from build123d import *

# Parameters (mm, degrees)
SKETCH_1_R          = 52.5
SKETCH_1_R_2        = 48.5
EXTRUDE_1_DEPTH     = 3.2
SKETCH_2_R          = 51.5
CUT_EXTRUDE_1_DEPTH = 2.2
SKETCH_3_R          = 1.25
EXTRUDE_2_DEPTH     = 1.1
EXTRUDE_3_DEPTH     = 1.1
SKETCH_5_R          = 0.7
CUT_EXTRUDE_2_DEPTH = 75.315139776
SKETCH_6_R          = 1.5
CUT_EXTRUDE_3_DEPTH = 0.7
FILLET_1_R          = 0.5
CHAMFER_1_SIZE      = 0.3
CHAMFER_1_SIZE2     = 0.357526078


with BuildPart() as part:
    # 草图1 → 凸台-拉伸1 (new body)
    with BuildSketch(Plane(origin=(0, 0, 0), x_dir=(1, 0, 0), z_dir=(0, 1, 0))):
        with Locations(Location((0, 0, 0), (0, 0, 270))):
            Circle(SKETCH_1_R)
        with Locations(Location((0, 0, 0), (0, 0, 270))):
            Circle(SKETCH_1_R_2, mode=Mode.SUBTRACT)
    extrude(amount=EXTRUDE_1_DEPTH)

    # 草图2 → 切除-拉伸1 (cut)
    with BuildSketch(Plane(origin=(0, 3.2, 0), x_dir=(1, 0, 0), z_dir=(0, 1, 0))):
        with Locations(Location((0, 0, 0), (0, 0, 270))):
            Circle(SKETCH_2_R)
    extrude(amount=-CUT_EXTRUDE_1_DEPTH, mode=Mode.SUBTRACT)

    # 草图3 → 凸台-拉伸2 (add)
    with BuildSketch(Plane(origin=(0, 1, 0), x_dir=(1, 0, 0), z_dir=(0, 1, 0))):
        with Locations((-43.734282891, -25.25)):
            Circle(SKETCH_3_R)
        with Locations((43.734282891, -25.25)):
            Circle(SKETCH_3_R)
        with Locations((0, 50.5)):
            Circle(SKETCH_3_R)
    extrude(amount=EXTRUDE_2_DEPTH)

    # 草图4 → 凸台-拉伸3 (add)
    with BuildSketch(Plane(origin=(0, 1, 0), x_dir=(1, 0, 0), z_dir=(0, 1, 0))):
        with BuildLine():
            ThreePointArc((-44.974169566, -25.09131467), (-44.774871009, -24.557413277), (-44.359282891, -24.167468245))
            Line((-44.359282891, -24.167468245), (-45.225308295, -24.667468245))
            Line((-45.225308295, -24.667468245), (-44.600307976, -25.750000552))
            ThreePointArc((-44.600307976, -25.750000552), (-44.788449666, -25.4213449), (-44.974169566, -25.09131467))
        make_face()
        with BuildLine():
            Line((-43.975308295, -26.832531755), (-43.109282891, -26.332531755))
            ThreePointArc((-43.109282891, -26.332531755), (-43.654779254, -26.497469106), (-44.216800701, -26.403116023))
            ThreePointArc((-44.216800701, -26.403116023), (-44.409754992, -26.077263307), (-44.600307976, -25.750000552))
            Line((-44.600307976, -25.750000552), (-43.975308295, -26.832531755))
        make_face()
        with BuildLine():
            Line((-1.59e-07, 51.5), (-1.25, 51.5))
            Line((-1.25, 51.5), (-1.25, 50.5))
            ThreePointArc((-1.25, 50.5), (-1.120091755, 51.054882384), (-0.757368864, 51.494430693))
            ThreePointArc((-0.757368864, 51.494430693), (-0.37869475, 51.498607654), (-1.59e-07, 51.5))
        make_face()
        with BuildLine():
            Line((1.25, 51.5), (-1.59e-07, 51.5))
            ThreePointArc((-1.59e-07, 51.5), (0.378694591, 51.498607655), (0.757368864, 51.494430693))
            ThreePointArc((0.757368864, 51.494430693), (1.120091755, 51.054882384), (1.25, 50.5))
            Line((1.25, 50.5), (1.25, 51.5))
        make_face()
        with BuildLine():
            Line((45.225308295, -24.667468245), (44.359282891, -24.167468245))
            ThreePointArc((44.359282891, -24.167468245), (44.774871009, -24.557413277), (44.974169566, -25.09131467))
            ThreePointArc((44.974169566, -25.09131467), (44.788449793, -25.421344676), (44.600308233, -25.750000108))
            Line((44.600308233, -25.750000108), (45.225308295, -24.667468245))
        make_face()
        with BuildLine():
            ThreePointArc((44.216800701, -26.403116023), (43.654779254, -26.497469107), (43.109282891, -26.332531755))
            Line((43.109282891, -26.332531755), (43.975308295, -26.832531755))
            Line((43.975308295, -26.832531755), (44.600308233, -25.750000108))
            ThreePointArc((44.600308233, -25.750000108), (44.409755121, -26.077263086), (44.216800701, -26.403116023))
        make_face()
    extrude(amount=EXTRUDE_3_DEPTH)

    # 草图5 → 切除-拉伸2 (cut, through all)
    with BuildSketch(Plane(origin=(0, 3.2, 0), x_dir=(1, 0, 0), z_dir=(0, 1, 0))):
        with Locations(Location((0, 50.5, 0), (0, 0, 270))):
            Circle(SKETCH_5_R)
        with Locations(Location((-43.734282891, -25.25, 0), (0, 0, 270))):
            Circle(SKETCH_5_R)
        with Locations(Location((43.734282891, -25.25, 0), (0, 0, 270))):
            Circle(SKETCH_5_R)
    extrude(amount=-CUT_EXTRUDE_2_DEPTH, mode=Mode.SUBTRACT)

    # 草图6 → 切除-拉伸3 (cut)
    with BuildSketch(Plane.XZ):
        with Locations(Location((-43.734282891, 25.25, 0), (0, 0, 270))):
            Circle(SKETCH_6_R)
        with Locations(Location((0, -50.5, 0), (0, 0, 270))):
            Circle(SKETCH_6_R)
        with Locations(Location((43.734282891, 25.25, 0), (0, 0, 270))):
            Circle(SKETCH_6_R)
    extrude(amount=-CUT_EXTRUDE_3_DEPTH, mode=Mode.SUBTRACT)

    # 圆角1
    fillet_1_edges = [part.edges().sort_by_distance(p)[0] for p in [
        (0, 0, -52.5),
        (-43.962168838, 1.55, 26.824945686),
        (-45.212168838, 1.55, 24.659882176),
        (-1.25, 1.55, -51.484827862),
        (1.25, 1.55, -51.484827862),
        (45.212168838, 1.55, 24.659882176),
        (43.962168838, 1.55, 26.824945686),
    ]]
    fillet(fillet_1_edges, radius=FILLET_1_R - 0.0001)  # a hair under: the kernel refuses the full size

    # 倒角1
    chamfer_1_edges = [part.edges().sort_by_distance(p)[0] for p in [
        (0, 0, -48.5),
    ]]
    chamfer_1_side = [part.faces().sort_by_distance(p)[0] for p in [
        (0, 0.5, -48.5),
    ]]
    chamfer(chamfer_1_edges, length=CHAMFER_1_SIZE, length2=CHAMFER_1_SIZE2, reference=chamfer_1_side[0])


solid = part.part
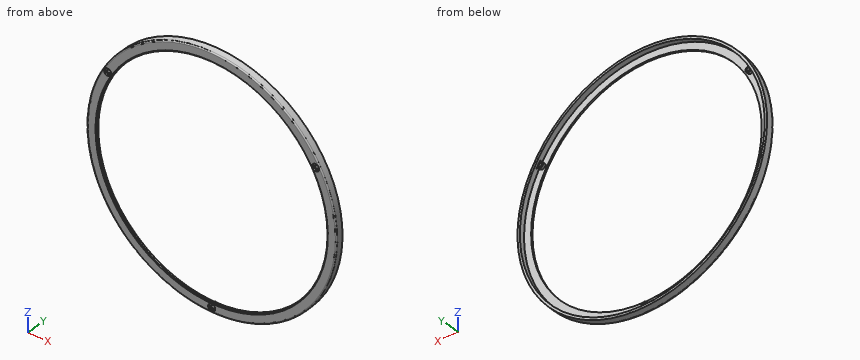
Read the model definition and answer for the solid it produces. Units are mm, in the model's axes. Coordinates: 2 decimals unless noted, no trailing zeros. Loops run counter-clockwise (first coordinate to the right, second up) from the corner with the lowest first, then second, coordinate; pieces in that order, holes last. Notation, with made-up numbers: (43, -16) - (92, -16) arc R25 ccw to (92, 5) - close; hole circle Ø5 at (61, 25.5). An arc over 180 degrees is marked (long way). Answer in a Markdown table with one row per item.
Q1. Given P1, Ø1.8, axis at x = 0.5, z = -50.5, coming from the +Y side; P2, Ø1, axis at y = 1, z = -24.5, coming from the -X side; P3, Ø1.5, axis at y = 0.5, z = -9.5, coming from the -X side, each flat-ended and moving along its own axis, determine where each tip first touches the part or whether it passes through.
Here are the results:
| item | result |
|---|---|
| P1 | stops at y = 2.1 |
| P2 | stops at x = -46.69 |
| P3 | stops at x = -51.77 |
Q2. Find section B-B on y = 1.6. Write down the section's boundary in (x, z).
Here are the results:
| item | result |
|---|---|
| outline | circle Ø105 at (0, 0); hole (-45.46, 24.2) arc R51.5 ccw to (-1.77, -51.47) arc R0.5 ccw to (-1.25, -50.97) - (-1.25, -50.5) arc R1.25 cw to (1.25, -50.5) - (1.25, -50.97) arc R0.5 ccw to (1.77, -51.47) arc R51.5 ccw to (45.46, 24.2) arc R0.5 ccw to (44.77, 24.4) - (44.36, 24.17) arc R1.25 cw to (43.11, 26.33) - (43.52, 26.57) arc R0.5 ccw to (43.69, 27.27) arc R51.5 ccw to (-43.69, 27.27) arc R0.5 ccw to (-43.52, 26.57) - (-43.11, 26.33) arc R1.25 cw to (-44.36, 24.17) - (-44.77, 24.4) arc R0.5 ccw to start; hole circle Ø1.4 at (-43.73, 25.25); hole circle Ø1.4 at (0, -50.5); hole circle Ø1.4 at (43.73, 25.25) |
Q3. Straight lines are drawn through the part: line 1 along X through (y, z) = (0.4, 25.25); line 2 along Z through (x, y) = (-0.5, 1.6); line 3 along X through (y, z) = (1.45, -18.5). For each, find the intervals that lie inside material, in ascending order. Write a range as [from, to].
Here are the results:
| item | result |
|---|---|
| line 1 | x = [-46.02, -45.23], [-42.23, -41.41], [41.41, 42.23], [45.23, 46.02] |
| line 2 | z = [-52.5, -50.99], [-50.01, -49.35], [51.5, 52.5] |
| line 3 | x = [-49.13, -48.06], [48.06, 49.13] |
Q4. Find section A-A on z = 0. Write down the section's boundary in (x, y).
Here are the results:
| item | result |
|---|---|
| outline | (-52.5, 0.5) arc R0.5 ccw to (-52, 0) - (-48.86, 0) - (-48.5, 0.3) - (-48.5, 1) - (-51.5, 1) - (-51.5, 3.2) - (-52.5, 3.2) - close; (48.5, 0.3) - (48.86, 0) - (52, 0) arc R0.5 ccw to (52.5, 0.5) - (52.5, 3.2) - (51.5, 3.2) - (51.5, 1) - (48.5, 1) - close |
